```python
from build123d import *

# Parameters (mm, degrees)
SKETCH1_R                 = 12.7
BASE_EXTRUDE_DEPTH        = 16.5
SKETCH4_R                 = 1.1303
CUT_EXTRUDE1_DEPTH        = 38.570999454
F_8_32_TAPPED_HOLE1_D     = 3.4544
F_8_32_TAPPED_HOLE1_DEPTH = 6.35
F_8_32_TAPPED_HOLE1_TIP   = 1.037806461
CUT_EXTRUDE2_REACH        = 34.844
CUT_EXTRUDE2_END_RADIUS   = 1.1303
SKETCH9_R                 = 1.1303
SKETCH10_W                = 27.33350128
SKETCH10_H                = 0.25
CUT_EXTRUDE3_DEPTH        = 0.25
SKETCH11_R                = 0.5
CUT_EXTRUDE4_DEPTH        = 25.389137098


with BuildPart() as part:
    # Sketch1 → Base-Extrude (new, symmetric)
    with BuildSketch(Plane.XY):
        Circle(SKETCH1_R)
    extrude(amount=BASE_EXTRUDE_DEPTH, both=True)

    # Sketch2 → 1/4-20 Tapped Hole1 (revolve, cut)
    with BuildSketch(Plane(origin=(0, 0, 16.5), x_dir=(0, -1, 0), z_dir=(1, 0, 0))):
        Polygon((0, 0), (0, 7.883816902), (2.5527, 6.35), (2.5527, 0), align=None)
    f_1_4_20_tapped_hole1 = revolve(axis=Axis((0, 0, 22.85), (0, 0, -1)), mode=Mode.SUBTRACT)

    # Mirror1: 1/4-20 Tapped Hole1 across plane
    add(f_1_4_20_tapped_hole1.mirror(Plane.XY), mode=Mode.SUBTRACT)

    # Sketch4 → Cut-Extrude1 (cut, through all)
    with BuildSketch(Plane.XY.offset(16.5)):
        Circle(SKETCH4_R)
    extrude(amount=-CUT_EXTRUDE1_DEPTH, mode=Mode.SUBTRACT)

    # #8-32 Tapped Hole1
    with Locations(Plane(origin=(12.7, 0, 0), x_dir=(0, 0, -1), z_dir=(1, 0, 0))):
        with Locations((0, 0)):
            Hole(F_8_32_TAPPED_HOLE1_D / 2, depth=F_8_32_TAPPED_HOLE1_DEPTH)
            with Locations((0, 0, -(F_8_32_TAPPED_HOLE1_DEPTH + F_8_32_TAPPED_HOLE1_TIP / 2))):  # 118° drill point
                Cone(0, F_8_32_TAPPED_HOLE1_D / 2, F_8_32_TAPPED_HOLE1_TIP, mode=Mode.SUBTRACT)

    # Cut-Extrude2: up to this cylinder (the profile starts outside it)
    cut_extrude2_end = Plane(origin=(0, 0, 0), z_dir=(0, 0, 1)) * Cylinder(CUT_EXTRUDE2_END_RADIUS, 72.9486, mode=Mode.PRIVATE)
    # Sketch9 → Cut-Extrude2 (cut, up to the surface)
    with BuildSketch(Plane(origin=(12.7, 0, 0), x_dir=(0, 0, -1), z_dir=(1, 0, 0)), mode=Mode.PRIVATE) as cut_extrude2_sk1:
        Circle(SKETCH9_R)
    cut_extrude2_tool1 = extrude(cut_extrude2_sk1.sketch, amount=-CUT_EXTRUDE2_REACH, mode=Mode.PRIVATE) - cut_extrude2_end
    add(cut_extrude2_tool1.solids().sort_by_distance((12.7, 0, 0))[0], mode=Mode.SUBTRACT)

    # Sketch10 → Cut-Extrude3 (cut)
    with BuildSketch(Plane.XY.offset(16.5)):
        with Locations((0.215070468, 0)):
            Rectangle(SKETCH10_W, SKETCH10_H)
    cut_extrude3 = extrude(amount=-CUT_EXTRUDE3_DEPTH, mode=Mode.SUBTRACT)

    # Mirror2: Cut-Extrude3 across plane
    add(cut_extrude3.mirror(Plane.XY), mode=Mode.SUBTRACT)

    # Sketch11 → Cut-Extrude4 (cut, through all)
    with BuildSketch(Plane(origin=(0, 0, 0), x_dir=(1, 0, 0), z_dir=(0, 1, 0))):
        with Locations(Location((0, 0, 0), (0, 0, 90))):
            Circle(SKETCH11_R)
    extrude(amount=CUT_EXTRUDE4_DEPTH, mode=Mode.SUBTRACT)


solid = part.part
```
Here's how the part is built. I have some questions about the finished solid (model axes, mm). A direction names the side the tool comes from. Coordinates: 2 decimals unless noted, no trailing zeros. Loops run counter-clockwise (first coordinate to the right, second up) from the corner with the lowest first, then second, coordinate; pieces in that order, holes last. Notation, with made-up numbers: (63, 85) - (98, 85) arc R7 cw to (98, 98) - close; hole circle Ø1 at (-26.5, -10). An arc over 180 degrees is marked (long way). Return JSON: item names as keys, results as strings. Group by question number.
Item 1: If we section it at C-C on y = 3.5: Write out the boundary of the cut face in (x, z).
Item 2: If we section it at D-D on x = -11: Write out the boundary of the cut face in (y, z) (3 decimals).
Item 3: We'd pull the mould along X, two halves only. Please class faces 1 (the face through (-2.75, -12.4, 0.23)), 2 (the face through (3.703, -0.688, 0.897)), 3 (the face through (-0.897, -0.688, 0.13)): +X half, -X half, draft (parallel to the pull), parting line (faces both ways), or undercut.
Item 4: Will these pins go through, and if not, where does the flat tip stop? P1, Ø8, axis at y = 7, z = -7, coming from the -X side; P2, Ø1, axis at y = 8, z = 3.5, coming from the +X side; P3, Ø2.5, axis at x = 0, y = 0, coming from the +Z side.
Item 5: If we section it at A-A on z = -6.5: Write out the boundary of the cut face in (x, y).
Item 6: If we section it at B-B on x = 4: Write out the boundary of the cut face in (y, z) (3 decimals), and give its area (3 significant figures).
Item 7: On a 3-axis mill with a long thin cutter (end or side, diameter ignored), from which of +Z, -Z, +X, -X, +Y, -Y can I reach the whole of each face in a straight line? I mean faces 4 (the face through (9.481, 1.713, -0.225)), 5 (the face through (-0.767, -2.435, -13.369)), 6 (the face through (0.488, 6.775, 0.108)), 7 (the face through (-0.767, -2.435, 13.369)). Say none if no direction works.
Item 8: I need wall thicknesses on line 1 (X direction, y = 0, z = -13); line 2 (Z direction, x = 2, y = 1). Which ranges of each line are inside material? Lowest first, please. Write a range as from..to.
Calculated:
{
 "1": {"outline": "(-12.21, -16.5) - (12.21, -16.5) - (12.21, 16.5) - (-12.21, 16.5) - close; hole circle Ø1 at (0, 0)"},
 "2": {"outline": "(-6.347, -16.5) - (-0.125, -16.5) - (-0.125, -16.25) - (0.125, -16.25) - (0.125, -16.5) - (6.347, -16.5) - (6.347, 16.5) - (0.125, 16.5) - (0.125, 16.25) - (-0.125, 16.25) - (-0.125, 16.5) - (-6.347, 16.5) - close"},
 "3": {"face 1": "parting line", "face 2": "draft", "face 3": "undercut"},
 "4": {"P1": "stops at x = -12.34", "P2": "stops at x = 10.25", "P3": "stops at z = 9.37"},
 "5": {"outline": "circle Ø25.4 at (0, 0); hole circle Ø2.26 at (0, 0)"},
 "6": {"outline": "(-12.054, -16.5) - (-0.125, -16.5) - (-0.125, -16.25) - (0.125, -16.25) - (0.125, -16.5) - (12.054, -16.5) - (12.054, 16.5) - (0.125, 16.5) - (0.125, 16.25) - (-0.125, 16.25) - (-0.125, 16.5) - (-12.054, 16.5) - close; hole circle Ø2.261 at (0, 0)", "area": "791 mm^2"},
 "7": {"face 4": "+X", "face 5": "-Z", "face 6": "+Y", "face 7": "+Z"},
 "8": {"line 1": "x = -12.7..-2.55, 2.55..12.7", "line 2": "z = -9.96..-0.53, 0.53..9.96"}
}
